Geometry: final body of the model. Coordinates: model frame, mm. Face numbers are marked on the shaded views. A direction names the side the tool comes from. Give positions to 0.01 mm unless a question says otherwise; leave off trailing zeros. Loops run counter-clockwise (first coordinate to the right, second up) from the corner with the lowest first, then second, coordinate; pieces in that order, holes last. Notation, with made-up numbers: (-0.75, 10) - (57.25, 10) arc R23 cw to (57.25, 48) - close; hole circle Ø9 at (15, 15.5). An arc over 180 degrees is marked (long way). Use CSV: the item, a comma, the result in double quotes. Start each with the question number.
```python
from build123d import *

# Parameters (mm, degrees)
SKETCH_R     = 12.05
PAD_DEPTH    = 8.5
SKETCH003_W  = 36
SKETCH003_H  = 10
POCKET_DEPTH = 5.5


with BuildPart() as part:
    # Sketch → Pad (new body)
    with BuildSketch(Plane.XY):
        Circle(SKETCH_R)
    extrude(amount=PAD_DEPTH)

    # Sketch002 (on Face3 of Pad) → AdditiveLoft section 0
    with BuildSketch(Plane.XY.offset(8.5)):
        with BuildLine():
            ThreePointArc((-10.96369, 5), (-12.05, 0), (-10.96369, -5))
            Line((10.96369, -5), (-10.96369, -5))
            ThreePointArc((10.96369, -5), (12.05, 0), (10.96369, 5))
            Line((-10.96369, 5), (10.96369, 5))
        make_face()
    # Sketch003 → AdditiveLoft section 1
    with BuildSketch(Plane.XY.offset(33.3)):
        Rectangle(SKETCH003_W, SKETCH003_H)
    loft()

    # Sketch004 (on Face2 of AdditiveLoft) → Pocket (cut)
    with BuildSketch(Plane(origin=(0, 0, 0), x_dir=(1, 0, 0), z_dir=(0, 0, -1))):
        Polygon((-3.781644, 6.55), (-7.563289, 0), (-3.781644, -6.55), (3.781644, -6.55), (7.563289, 0), (3.781644, 6.55), align=None)
    extrude(amount=-POCKET_DEPTH, mode=Mode.SUBTRACT)


solid = part.part
```
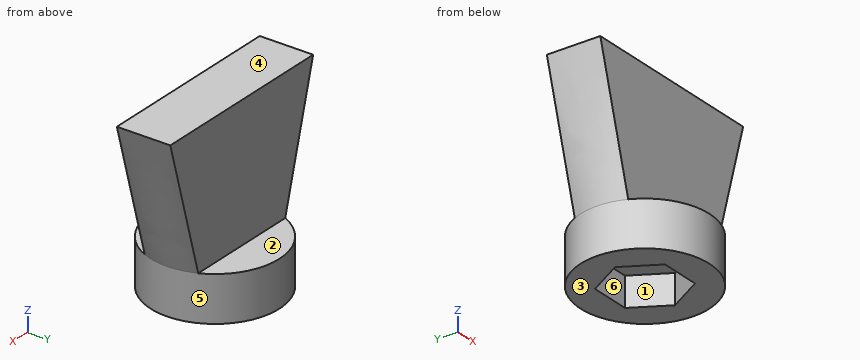
Item 1: Reachability of the marked faces 1, 2 and 3 from +Z, -Z, +X, -X, +Y, -Y: full face, straight path, thin tool, end or side. Return the list, or none.
Item 2: Section A-A (y = -8). Output: boundary loops of the cut face in (x, z), plus the area to 3 significant figures.
Item 3: Ray query, probe 1 along Y at (x, z) = (-4, 23.5); probe 2 along Z at (x, y) = (5.5, -10.5); probe 3 along X at (y, z) = (-1, 18). Return the intervals inside material, ascending.
Item 4: Mould query, pull axis Y, two halves, no side actions, for the marked faces 4, 5 and 6. Classes: pulls with the +Y half, pulls with the -Y half, needs draft (parallel to the pull), parting line crosses it, or undercut.
Item 5: Pin query (flat end, axial travel): pin 1 Ø3.5 at (x, y) = (2.5, -7.5) entering from +Z; pin 2 Ø4 at (y, z) = (1, 8.5) entering from -X; pin 3 Ø3 at (x, y) = (5, 5.5) entering from -Z; pin 4 Ø6 at (x, z) = (-6, 12) entering from +Y. Return the tip coordinate at first contact, or that it passes through.
Outcome:
1,face 1,"-Z"
1,face 2,"+Z, +X, -X, +Y"
1,face 3,"-Z, +X, -X, +Y, -Y"
2,outline,"(-9.01, 0) - (9.01, 0) - (9.01, 8.5) - (-9.01, 8.5) - close"
2,area,"153 mm2"
3,probe 1,"y = -5 to 5"
3,probe 2,"z = 0 to 8.5"
3,probe 3,"x = -14.3 to 14.3"
4,face 4,"needs draft"
4,face 5,"parting line crosses it"
4,face 6,"undercut"
5,pin 1,"stops at z = 8.5"
5,pin 2,"stops at x = -12.51"
5,pin 3,"stops at z = 0"
5,pin 4,"stops at y = 5"
